For this review, take the finished solid that the model builds, in its own axes (mm). Face numbers are marked on the shaded views. A direction names the side the tool comes from. Coordinates: 2 decimals unless noted, no trailing zeros. Write each loop counter-clockwise with the first axis right and the second up, starting at its lowest first coordinate (ties: lowest second). Pieces come first, ordered by that corner, then holes.
1) Mouldability with a two-part tool opening along X and no side actions: class the marked faces 1, 2 and 3 as pulls with the +X half, pulls with the -X half, needs draft (parallel to the pull), parting line crosses it, or undercut.
2) We need section B-B on z = -21. Write out the cut boundary in (x, y).
3) For the marked faces 4 and 5, list the 3-axis set-ups (+Z, -Z, +X, -X, +Y, -Y) from which the entire face can be reached by the end or side of a thin tool; tool diameter is ignored.
4) We need section D-D on y = -10.5. Give the number of separate pieces and of enclosed holes in the cut face, then the cut area to 3 significant figures.
5) To check wall thickness, follow line 1 along Z through (x, y) = (-84.9, -6.35) (3 decimals); line 2 along X through (y, z) = (-4.5, -47); line 3 along Z through (x, y) = (75.25, -6.35) (3 decimals). State the ranges of each line that lie inside material, in increasing order.
6) Insertion check: P1, Ø6, axis at y = -9, z = 28.5, coming from the +X side; P2, Ø4, axis at y = -8, z = 2.5, coming from the -X side; P3, Ø6.5, axis at y = -6.5, z = 44, coming from the +X side; P4, Ø1.4, axis at y = -6, z = 45, coming from the -X side. Each pin has a flat end and moves straight along its axis. Give the tip position at first contact, or say it passes through.
7) We need section A-A on x = -73.5. Write out the cut boundary in (y, z) (3 decimals).
8) We need section C-C on x = 15.5. Write out the cut boundary in (y, z) (3 decimals).
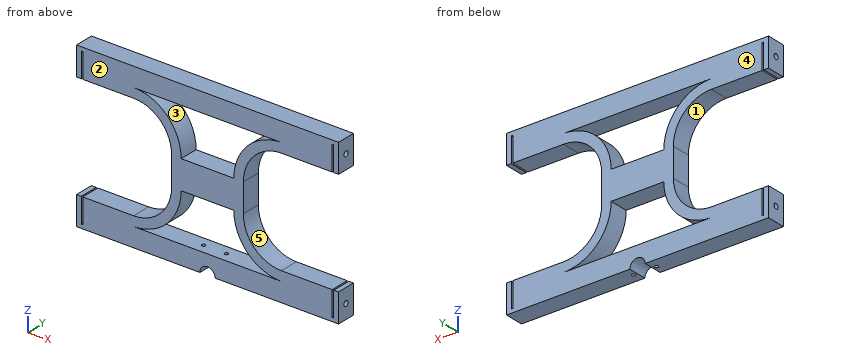
from build123d import *

# Parameters (mm, degrees)
F1_DEPTH  = 12.7
F2_W      = 1.016
F2_H      = 102.87
F3_DEPTH  = 25.4
F4_R      = 5.08
F5_DEPTH  = 25.4
F6_R      = 1.21539
F7_DEPTH  = 25.4
F8_R      = 1.397
F9_DEPTH  = 25.4
F10_R     = 1.397
F11_DEPTH = 19.05
F12_R     = 1.778
F13_DEPTH = 3.175
F15_DEPTH = 25.4
F16_W     = 12.7
F16_H     = 19.05
F17_DEPTH = 38.1


# Not quite as in the source:
# - a pattern or mirror of a feature is missing from the dataset's text; its kind, count and spacing are read off the source's solid


with BuildPart() as f1:
    # F0 (on Front) → F1 (new body)
    with BuildSketch(Plane.XZ):
        with BuildLine():
            Line((87.4268, 34.925), (87.4268, 53.975))
            Line((87.4268, 53.975), (0, 53.975))
            Line((0, 53.975), (-87.4268, 53.975))
            Line((-87.4268, 53.975), (-87.4268, 34.925))
            Line((-87.4268, 34.925), (-49.3268, 34.925))
            ThreePointArc((-49.3268, 34.925), (-31.3662877579, 27.4855122421), (-23.9268, 9.525))
            Line((-23.9268, 9.525), (-23.9268, -9.525))
            ThreePointArc((-23.9268, -9.525), (-31.3662877579, -27.4855122421), (-49.3268, -34.925))
            Line((-49.3268, -34.925), (-87.4268, -34.925))
            Line((-87.4268, -34.925), (-87.4268, -53.975))
            Line((-87.4268, -53.975), (87.4268, -53.975))
            Line((87.4268, -53.975), (87.4268, -34.925))
            Line((87.4268, -34.925), (49.3268, -34.925))
            ThreePointArc((49.3268, -34.925), (31.3662877579, -27.4855122421), (23.9268, -9.525))
            Line((23.9268, -9.525), (23.9268, 9.525))
            ThreePointArc((23.9268, 9.525), (31.3662877579, 27.4855122421), (49.3268, 34.925))
            Line((49.3268, 34.925), (87.4268, 34.925))
        make_face()
    extrude(amount=F1_DEPTH)

    # F2 (on face) → F3 (cut)
    with BuildSketch(Plane.XZ.offset(12.7)):
        with Locations((-83.7438, 0)):
            Rectangle(F2_W, F2_H)
        with Locations((83.7438, 0)):
            Rectangle(F2_W, F2_H)
    extrude(amount=-F3_DEPTH, mode=Mode.SUBTRACT)

    # F4 (on face) → F5 (cut)
    with BuildSketch(Plane.XZ.offset(12.7)):
        with Locations((0, -53.975)):
            Circle(F4_R)
    extrude(amount=-F5_DEPTH, mode=Mode.SUBTRACT)

    # F6 (on face) → F7 (cut)
    with BuildSketch(Plane(origin=(0, 0, -53.975), x_dir=(1, 0, 0), z_dir=(0, 0, -1))):
        with Locations((-7.62, 6.35)):
            Circle(F6_R)
        with Locations((7.62, 6.35)):
            Circle(F6_R)
    extrude(amount=-F7_DEPTH, mode=Mode.SUBTRACT)

    # F8 (on face) → F9 (cut)
    with BuildSketch(Plane.YZ.offset(87.4268)):
        with Locations((-6.35, 44.45)):
            Circle(F8_R)
        with Locations((-6.35, -44.45)):
            Circle(F8_R)
    extrude(amount=-F9_DEPTH, mode=Mode.SUBTRACT)

    # F10 (on face) → F11 (cut)
    with BuildSketch(Plane(origin=(-87.4268, 0, 0), x_dir=(0, -1, 0), z_dir=(-1, 0, 0))):
        with Locations((6.35, 44.45)):
            Circle(F10_R)
        with Locations((6.35, -44.45)):
            Circle(F10_R)
    extrude(amount=-F11_DEPTH, mode=Mode.SUBTRACT)

    # F12 (on face) → F13 (cut)
    with BuildSketch(Plane.YZ.offset(87.4268)):
        with Locations((-6.35, 44.45)):
            Circle(F12_R)
        with Locations((-6.35, -44.45)):
            Circle(F12_R)
    f13 = extrude(amount=-F13_DEPTH, mode=Mode.SUBTRACT)

    # F13_copies: F13 across plane
    add(f13.mirror(Plane(origin=(0, 0, 0), x_dir=(0, 0, -1), z_dir=(-1, 0, 0))), mode=Mode.SUBTRACT)

    # F14 (on face) → F15 (cut)
    with BuildSketch(Plane.XZ.offset(12.7)):
        with BuildLine():
            ThreePointArc((-17.5768, -9.525), (-26.8761596973, -31.9756403027), (-49.3268, -41.275))
            Line((-49.3268, -41.275), (49.3268, -41.275))
            ThreePointArc((49.3268, -41.275), (26.8761596973, -31.9756403027), (17.5768, -9.525))
            Line((17.5768, -9.525), (17.5768, 9.525))
            ThreePointArc((17.5768, 9.525), (26.8761596973, 31.9756403027), (49.3268, 41.275))
            Line((49.3268, 41.275), (-49.3268, 41.275))
            ThreePointArc((-49.3268, 41.275), (-26.8761596973, 31.9756403027), (-17.5768, 9.525))
            Line((-17.5768, 9.525), (-17.5768, -9.525))
        make_face()
    extrude(amount=-F15_DEPTH, mode=Mode.SUBTRACT)

    # F16 (on face) → F17 (join)
    with BuildSketch(Plane.YZ.offset(-17.5768)):
        with Locations((-6.35, 0)):
            Rectangle(F16_W, F16_H)
    extrude(amount=F17_DEPTH)


solid = f1.part
Result:
1. face 1: pulls with the -X half
1. face 2: needs draft
1. face 3: undercut
2. outline: (-26.67, -12.7) - (-19.72, -12.7) - (-19.72, 0) - (-26.67, 0) - close; (19.72, -12.7) - (26.67, -12.7) - (26.67, 0) - (19.72, 0) - close
3. face 4: +Z, -Z, +X, -X, +Y
3. face 5: +X, +Y, -Y
4. separate pieces: 1
4. enclosed holes: 2
4. area: 7,350 mm2
5. line 1: z = -53.975 to -46.228, -42.672 to -34.925, 34.925 to 42.672, 46.228 to 53.975
5. line 2: x = -87.43 to -84.25, -83.24 to 83.24, 84.25 to 87.43
5. line 3: z = -53.975 to -45.847, -43.053 to -34.925, 34.925 to 43.053, 45.847 to 53.975
6. P1: stops at x = 36.59
6. P2: stops at x = -23.93
6. P3: stops at x = 87.43
6. P4: stops at x = -68.38
7. outline: (-12.7, -53.975) - (0, -53.975) - (0, -34.925) - (-12.7, -34.925) - close; (-12.7, 34.925) - (0, 34.925) - (0, 53.975) - (-12.7, 53.975) - close; hole circle Ø2.794 at (-6.35, -44.45); hole circle Ø2.794 at (-6.35, 44.45)
8. outline: (-12.7, -53.975) - (0, -53.975) - (0, -41.275) - (-12.7, -41.275) - close; (-12.7, -9.525) - (0, -9.525) - (0, 9.525) - (-12.7, 9.525) - close; (-12.7, 41.275) - (0, 41.275) - (0, 53.975) - (-12.7, 53.975) - close
